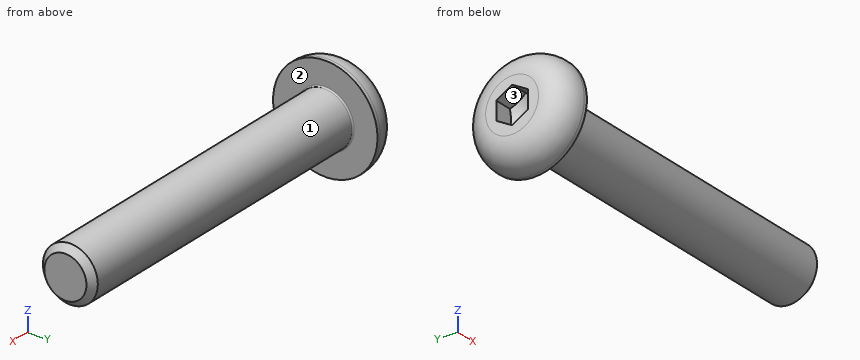
Autodesk Inventor part; units mm, degrees
ref_plane "Work Plane1" through (29, 0, 0) normal (0, -1, 0) x (1, 0, 0)
ref_plane "YZ Plane" through (0, 0, 0) normal (1, 0, 0) x (0, 1, 0)
ref_plane "XZ Plane" through (0, 0, 0) normal (0, 1, 0) x (-1, 0, 0)
sketch "Sketch1" plane through (0, 0, 0) normal (0, 0, 1) x (1, 0, 0)
  line L0 (-0.0931, 0) -> (25.4, 0)
  line L1 (25.4, 0) -> (25.4, 2.0828)
  line L2 (25.4, 2.0828) -> (1.5902, 2.0828)
  line L3 (1.5902, 2.0828) -> (0.0001, 2.0828)
  line L4 (0.0001, 2.0828) -> (0, 2.0828)
  line L5 (0, 2.0828) -> (0, 3.9624)
  line L6 (0, 3.9624) -> (-2.2098, 3.9624)
  line L7 (-2.2098, 3.9624) -> (-2.2098, 1.3785)
  line L8 (-2.2098, 1.3785) -> (-0.889, 1.3785)
  line L9 (-0.889, 1.3785) -> (-0.0931, 0)
  line L10 (-7.7318, 0) -> (30.922, 0)
  line L11 (0, -0.7925) -> (0, 4.7549)
  line L12 (1.5902, 2.0828) -> (0, 2.0828) construction
  dimension "d1" = 23.8098
  dimension "d2" = 1.5901
  dimension "d3" = 2.2098
  dimension "d4" = 1.3208
  dimension "d5" = 60
  dimension "d6" = 4.1656
  dimension "d7" = 4.1656
  dimension "d8" = 2.757
  dimension "d9" = 7.9248
  dimension "d26" = 25.4
revolve "Body" add sketch "Sketch1" angle 360 about axis through (-0.0931, 0, 0) along (1, 0, 0)
sketch "Sketch2" plane through (-2.2098, 0, 0) normal (-1, 0, 0) x (0, 0, 1)
  circle A0 centre (0, 0) radius 1.3785
  line L0 (0, -5.5474) -> (0, 5.5474)
  line L1 (-5.5474, 0) -> (5.5474, 0)
  line L2 (1.3785, 0) -> (0.6892, -1.1938)
  line L3 (0.6892, -1.1938) -> (-0.6892, -1.1938)
  line L4 (-0.6892, -1.1938) -> (-1.3785, 0)
  line L5 (-1.3785, 0) -> (-0.6892, 1.1938)
  line L6 (-0.6892, 1.1938) -> (0.6892, 1.1938)
  line L7 (0.6892, 1.1938) -> (1.3785, 0)
extrude "Slot" add sketch "Sketch2" against normal up to next contours L7 A0 | A0 L2 | L6 L0 A0 | A0 L0 L3 | L0 L6 A0 | A0 L3 L0 | L4 A0 | A0 L5
fillet "Fillet1" radius 1.9558 1 edges at (-2.2098, -3.9624, 0)
thread "Thread"
chamfer "Chamfer1" distance 0.4869 distance2 0.4869 1 edges at (25.4, -2.0828, 0) measured on face at (25.4, -0.0273, 0.4604)
ref_plane "Work Plane1" through (29, 0, 0) normal (0, -1, 0) x (1, 0, 0)
fillet "Fillet2" radius 0.1 1 edges at (0.0001, -2.0828, 0)
equation "\"d1\" = GEL"
equation "\"d3\" = KOH"
equation "\"d4\" = INTI"
equation "\"d6\" = GD"
equation "\"d7\" = BDM"
equation "\"d8\" = 1.1547 * SW"
equation "\"d9\" = KOD"
equation "\"d26\" = NLG"
equation "\"d30\" = R"
equation "\"d17\" = RR"
equation "\"d13\" = GEL"
equation "\"d15\" = -0.5 * SPD + 0.5 * GD"
equation "\"d16\" = GUL"
equation "\"GD\" = NND"
equation "\"NLG\" = 25.4"
equation "\"GEL\" = 23.80976"
equation "\"KOD\" = 7.9248"
equation "\"KOH\" = 2.2098"
equation "\"INTI\" = 1.3208"
equation "\"GAL\" = 1.59004"
equation "\"GUL\" = 0.48692"
equation "\"BDM\" = NND"
equation "\"SW\" = 2.3876"
equation "\"RR\" = 1.9558"
equation "\"SPD\" = 3.19176"
equation "\"R\" = 0.1"
equation "\"TOA\" = 30deg"
equation "\"GD1\" = SPD"
equation "\"THREADDIA\" = 4.1656"
equation "\"KOH1\" = 0.381"
equation "\"NND\" = 4.1656"
equation "\"E0\" = 2.75768"
properties part number "ANSI B18.3 - 8 - 32 x 1" material "Steel, Mild"
Input: part model. Units: mm. Frame: model coordinates. Face numbers are marked on the shaded views. Round coordinates to 2 decimals unless told otherwise and drop trailing zeros. Order: outer loops, then holes, each group sorted by start corner. A loop starts at its lowest first (then second) coordinate and runs counter-clockwise, first axis right, second up.
1. Material intervals for line 1 (Y direction, x = 20.25, z = 0); line 2 (X direction, y = -1, z = -0.25); line 3 (Z direction, x = -0.75, y = 0.5), sorted ascending.
The answers:
line 1: y = -2.08 to 2.08
line 2: x = -0.69 to 25.4
line 3: z = -3.87 to -1.02, 1.02 to 3.87
2. Pin query (flat end, axial travel): P1, Ø1.1, axis at x = -1.5, z = -0.5, coming from the -Y side; P2, Ø1.5, axis at x = 4, y = 2, coming from the -Z side; P3, Ø0.7, axis at x = -1.5, z = -0.5, coming from the +Y side. Return the tip coordinate at first contact, or that it passes through.
The answers:
P1: stops at y = -3.81
P2: stops at z = -1.67
P3: stops at y = 3.72
3. Cut plane A-A, the plane x = 6. Output: boundary loops of the cut face in (y, z).
The answers:
outline: circle Ø4.17 at (0, 0)
4. Mould query, pull axis Z, two halves, no side actions, for the marked faces 1, 2 and 3. Classes: released by +Z, released by -Z, zero draft, split by the parting line, or undercut.
The answers:
face 1: split by the parting line
face 2: zero draft
face 3: undercut
